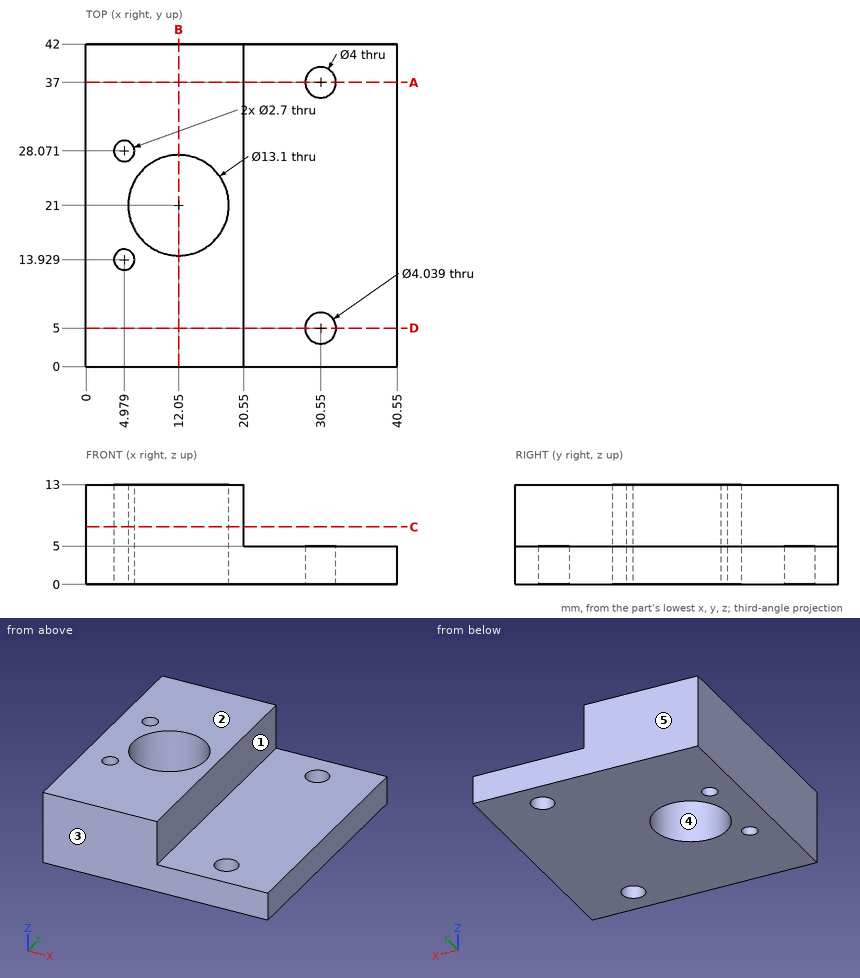
Geometry check sheet. Reference: drawing and pictorial views, mm from the part's lowest x, y, z. A direction names the side the tool comes from. Give positions to 0.01 mm unless a question says otherwise; leave off trailing zeros. Order: outer loops, then holes, each group sorted by start corner. A loop starts at its lowest first (then second) coordinate and runs counter-clockwise, first axis right, second up. Notation, with made-up numbers: (-13, -29.75) -> (2, -29.75) arc R32 cw to (2, 5.25) -> close; hole circle Ø6 at (25, -2). An arc over 180 degrees is marked (long way). Write each question's results on one line, items separated by ' | '. Start each with the question number.
(1) Scan lines: line 1 (Y direction, x = 30.55, z = 2.05); line 2 (Y direction, x = 12.05, z = 8.5); line 3 (Z direction, x = 33.5, y = 13). Record each from-to range of solid material in increasing order.
(2) Sectioned sample at D-D (y = 5). Enter the section's corners in (x, z), plus the area to 3 significant figures.
(3) Mould release check, pull along Y, two halves, no side actions. Record for the marked faces 3, 4 and 5: pulls with the +Y half, pulls with the -Y half, needs draft (parallel to the pull), parting line crosses it, or undercut.
(4) Gauge pin test, flat ends, axial feed: P1, Ø1.5, axis at y = 9, z = 8.5, coming from the +X side; P2, Ø5.5, axis at x = 30.55, y = 5, coming from the +Z side; P3, Ø12, axis at x = 12.05, y = 21, coming from the +Z side. Record the tip position at first contact, or that the pin passes through.
(5) Sectioned sample at C-C (z = 7.5). Enter the section's corners in (x, y), plus the area to 3 significant figures.
(6) Sectioned sample at B-B (x = 12.05). Enter the section's corners in (y, z).
(7) Sectioned sample at A-A (y = 37). Enter the section's corners in (x, z), plus the area to 3 significant figures.
(8) Access from +Z, -Z, +X, -X, +Y, -Y to the whole of each face (thin tool, end or side, straight path). Record for the marked faces 1 and 2.
Answer below:
1) line 1: 0 to 2.98, 7.02 to 35, 39 to 42 | line 2: 0 to 14.45, 27.55 to 42 | line 3: 0 to 5
2) outline: (0, 0) -> (28.53, 0) -> (28.53, 5) -> (20.55, 5) -> (20.55, 13) -> (0, 13) -> close; (32.57, 0) -> (40.55, 0) -> (40.55, 5) -> (32.57, 5) -> close | area: 347 mm2
3) face 3: pulls with the -Y half | face 4: undercut | face 5: pulls with the +Y half
4) P1: x = 20.55 | P2: z = 5 | P3: through
5) outline: (0, 0) -> (20.55, 0) -> (20.55, 42) -> (0, 42) -> close; hole circle Ø2.7 at (4.98, 13.93); hole circle Ø2.7 at (4.98, 28.07); hole circle Ø13.1 at (12.05, 21) | area: 717 mm2
6) outline: (0, 0) -> (14.45, 0) -> (14.45, 13) -> (0, 13) -> close; (27.55, 0) -> (42, 0) -> (42, 13) -> (27.55, 13) -> close
7) outline: (0, 0) -> (28.55, 0) -> (28.55, 5) -> (20.55, 5) -> (20.55, 13) -> (0, 13) -> close; (32.55, 0) -> (40.55, 0) -> (40.55, 5) -> (32.55, 5) -> close | area: 347 mm2
8) face 1: +Z, +X, +Y, -Y | face 2: +Z, +X, -X, +Y, -Y
